For this review, take the finished solid that the model builds, in its own axes (mm). Face numbers are marked on the shaded views. Give positions to 0.01 mm unless a question says otherwise; leave off trailing zeros. Order: outer loops, then holes, each group sorted by start corner. A loop starts at its lowest first (then second) coordinate and runs counter-clockwise, first axis right, second up. Notation, with made-up numbers: (17, -10) - (55, -10) arc R9 cw to (55, 1) - close; hole circle Ø5 at (-38.5, 77). An arc over 180 degrees is marked (long way). Use a Markdown table: item, result. Add a question column.
1) Clearance check with flat-ended pins moving along their axes: P1, Ø3, axis at x = -8, y = 12.5, coming from the +Z side; P2, Ø8, axis at x = 0, z = 0, coming from the -Y side; P3, Ø1, axis at x = 7.5, y = 8.5, coming from the -Z side; P4, Ø1, axis at x = -12, z = 4.5, coming from the -Y side. State where each tip first meets the part, or that it passes through.
2) We need section B-B on y = 14.25. Write out the cut boundary in (x, z).
3) Mouldability with a two-part tool opening along Z and no side actions: class the marked faces 1, 2 and 3 as released by +Z, released by -Z, zero draft, split by the parting line, or undercut.
4) We need section C-C on y = 6.5. Write out the cut boundary in (x, z).
5) Wall thickness on L1, parallel to Z at x = 0, y = 11.5; L2, parallel to Z at x = 0, y = 4: over which ranges is each line inside the solid? List them lowest first.
Autodesk Inventor part; units mm, degrees
ref_plane "YZ Plane" through (0, 0, 0) normal (1, 0, 0) x (0, 1, 0)
ref_plane "XZ Plane" through (0, 0, 0) normal (0, 1, 0) x (-1, 0, 0)
ref_plane "XY Plane" through (0, 0, 0) normal (0, 0, 1) x (1, 0, 0)
sketch "Sketch1" plane through (0, 0, 0) normal (0, 1, 0) x (-1, 0, 0)
  circle A0 centre (0, 0) radius 5.1
  circle A1 centre (0, 0) radius 12.5
  dimension "d0" = 10.2
  dimension "d1" = 25
extrude "Extrusion1" add sketch "Sketch1" along normal blind 11.35
sketch "Sketch2" plane through (0, 11.35, 0) normal (0, 1, 0) x (1, 0, 0)
  circle A0 centre (0, 0) radius 12.5
  circle A1 centre (0, 0) radius 5.1
  circle A2 centre (0, 0) radius 17.5
  dimension "d4" = 35
extrude "Extrusion2" add sketch "Sketch2" along normal blind 7 contours A0 | A2
chamfer "Chamfer1" distance 0.5 angle 45 1 edges at (12.5, 0, 0)
chamfer "Chamfer2" distance 0.5 angle 45 1 edges at (-17.5, 18.35, 0)
properties part number "Ydre_bøsning_stempel_stang"
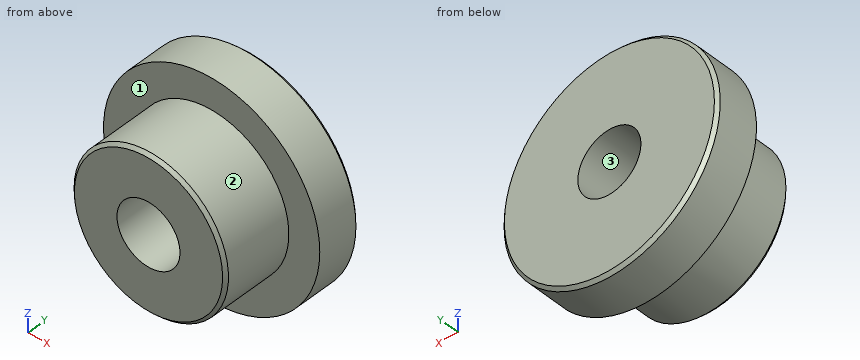
Checked values:
| question | item | result |
|---|---|---|
| 1 | P1 | z = 16.25 |
| 1 | P2 | through |
| 1 | P3 | z = -10.36 |
| 1 | P4 | y = 0.32 |
| 2 | outline | circle Ø35 at (0, 0); hole circle Ø10.2 at (0, 0) |
| 3 | face 1 | zero draft |
| 3 | face 2 | split by the parting line |
| 3 | face 3 | undercut |
| 4 | outline | circle Ø25 at (0, 0); hole circle Ø10.2 at (0, 0) |
| 5 | L1 | -17.5 to -5.1, 5.1 to 17.5 |
| 5 | L2 | -12.5 to -5.1, 5.1 to 12.5 |
